Verification items for the finished model (mm, model axes). A direction names the side the tool comes from. Round coordinates to 2 decimals unless told otherwise and drop trailing zeros. Write each loop counter-clockwise with the first axis right and the second up, starting at its lowest first coordinate (ties: lowest second). Pieces come first, ordered by that corner, then holes.
Autodesk Inventor part; units mm, degrees
ref_plane "YZ Plane" through (0, 0, 0) normal (1, 0, 0) x (0, 1, 0)
ref_plane "XZ Plane" through (0, 0, 0) normal (0, 1, 0) x (-1, 0, 0)
ref_plane "XY Plane" through (0, 0, 0) normal (0, 0, 1) x (1, 0, 0)
sketch "Sketch2" plane through (0, 0, 0) normal (0, 1, 0) x (-1, 0, 0)
  circle A0 centre (0, 0) radius 15
  dimension "d0" = 30
extrude "Extrusion1" add sketch "Sketch2" along normal blind 35
sketch "Sketch3" plane through (0, 35, 0) normal (0, 1, 0) x (1, 0, 0)
  circle A0 centre (0, 0) radius 3.6
  circle A1 centre (0, 0) radius 15
  circle A2 centre (0, 0) radius 10
  dimension "d3" = 7.2
  dimension "d4" = 20
extrude "Extrusion2" cut sketch "Sketch3" against normal blind 16 contours A1
extrude "Extrusion3" cut sketch "Sketch3" against normal blind 8 contours A2
sketch "Sketch4" plane through (0, 0, 0) normal (0, -1, 0) x (1, 0, 0)
  circle A0 centre (0, 0) radius 4.5
  dimension "d9" = 9
extrude "Extrusion4" cut sketch "Sketch4" against normal blind 7
properties part number "replacement-cover-axel"
Q1. Release check for a two-part mould opening along Z. For faces 4 (the cylindrical face through (3.434, 31.056, -1.081)), 5 (the flat face through (0, 7, 0)), 6 (the flat face through (3, 19, 10)) record: released by +Z, released by -Z, zero draft, split by the parting line, or undercut.
Recorded:
face 4: split by the parting line
face 5: undercut
face 6: zero draft
Q2. Material ranges on line 1 along Z through (x, y) = (0, 4); line 2 along Y through (x, z) = (7.5, -9.5); line 3 along Z through (x, y) = (-1.75, 2), recorded low to high.
Recorded:
line 1: z = -15 to -4.5, 4.5 to 15
line 2: y = 0 to 19
line 3: z = -14.9 to -4.15, 4.15 to 14.9
Q3. Sectioned sample at B-B (z = 0). Enter the section's corners in (x, y), plus the area to 3 significant figures.
Recorded:
outline: (-15, 0) - (-4.5, 0) - (-4.5, 7) - (4.5, 7) - (4.5, 0) - (15, 0) - (15, 19) - (10, 19) - (10, 27) - (3.6, 27) - (3.6, 35) - (-3.6, 35) - (-3.6, 27) - (-10, 27) - (-10, 19) - (-15, 19) - close
area: 725 mm2
Q4. Tool access check on faces 1 (the flat face through (4, 27, 0)), 2 (the cylindrical face through (-0.59, 3.45, 4.46)), 3 (the flat face through (0, 35, 0)). Record the directions out of +Z, -Z, +X, -X, +Y, -Y that give a thin tool (end or side, any length) a straight path to the whole face; none if there is none.
Recorded:
face 1: +Y
face 2: -Y
face 3: +Z, -Z, +X, -X, +Y
Q5. Sectioned sample at C-C (y = 3). Enter the section's corners in (x, z), plus the area to 3 significant figures.
Recorded:
outline: circle Ø30 at (0, 0); hole circle Ø9 at (0, 0)
area: 643 mm2
Q6. Sectioned sample at D-D (y = 16). Enter the section's corners in (x, z), plus the area to 3 significant figures.
Recorded:
outline: circle Ø30 at (0, 0)
area: 707 mm2
Q7. Sectioned sample at A-A (x = 0). Enter the section's corners in (y, z), plus the area to 3 significant figures.
Recorded:
outline: (0, -15) - (19, -15) - (19, -10) - (27, -10) - (27, -3.6) - (35, -3.6) - (35, 3.6) - (27, 3.6) - (27, 10) - (19, 10) - (19, 15) - (0, 15) - (0, 4.5) - (7, 4.5) - (7, -4.5) - (0, -4.5) - close
area: 725 mm2
Q8. Depth check by flat-ended pin: P1, Ø1, axis at x = -3, z = -3, coming from the +Y side; P2, Ø8, axis at y = 6.5, z = 11.5, coming from the -X side; P3, Ø1, axis at x = 3, y = 7, coming from the -Z side. Enter the tip coordinate at first touch or a pass-through.
Recorded:
P1: stops at y = 27
P2: stops at x = -12.99
P3: stops at z = -14.79
